Part model, mm, in its own coordinate system. A direction names the side the tool comes from. Coordinates: 2 decimals unless noted, no trailing zeros. Write each loop counter-clockwise with the first axis right and the second up, starting at its lowest first coordinate (ties: lowest second). Pieces come first, ordered by that corner, then holes. Notation, with made-up numbers: M 25,77 L 57,77 A14 cw 57,90 Z; hole C -7,86 d3. An arc over 180 degrees is marked long. Use a Markdown table: item, result. Add a question column.
Q1. Wall check: L1, parallel to X at y = -10.5, z = 0.5; L2, parallel to X at y = -56.9, z = -6; L3, parallel to Y at x = -12.5, z = 35.5. Give the ranges that are in metal, low to high. Write a range as from..to.
Q2. Mould opens along Y. For faces 6 (the flat face through (-39, -59, 9)), 7 (the flat face through (18.14, -46.86, 18.79)), 8 (the flat face through (12.606, 9, 2)), 9 (the flat face through (8.106, 9, 2)) say: released by +Y, released by -Y, zero draft, split by the parting line, or undercut.
Q3. Slice it at B-B on z = -6. Write the cut outline in (x, y), then the cut area to 3 significant figures.
Q4. Slice it at C-C on x = -11. Write the cut outline in (y, z).
Q5. Slice it at D-D on z = 29.5. Write the cut outline in (x, y), then the cut area to 3 significant figures.
Q6. Slice it at A-A on y = 1.5. Write the cut outline in (x, z).
Q7. Tool access for faces 1 (the flat face through (-4, -62.073, 29)), 2 (the flat face through (-4, -59, -15)), 3 (the flat face through (-22.394, 9, 2)), 4 (the flat face through (-5, -10, 0)), 5 (the cylindrical face through (-42.89, -59.59, -5.91)): list every direction of +Z, -Z, +X, -X, +Y, -Y with a clear straight run to the whole face (end or side of a thin tool).
Q8. Pin check, flat tips, straight feed: pin 1 Ø24 at (y, z) = (-48, 23.5) entering from -X; pin 2 Ø2 at (x, y) = (-15.5, 15.5) entering from +Z; pin 3 Ø12 at (x, y) = (11, -1.5) entering from -Z; pin 4 Ø6 at (y, z) = (-38.5, 18) entering from +X. Stop position of each tip, or through.
from build123d import *

# Parameters (mm, degrees)
ESQUISSE1_W             = 50
ESQUISSE1_H             = 95
BOSS_EXTRU_1_DEPTH      = 4
ESQUISSE2_W             = 50
ESQUISSE2_H             = 4
BOSS_EXTRU_2_DEPTH      = 5
ESQUISSE3_W             = 50
ESQUISSE3_H             = 5
BOSS_EXTRU_3_DEPTH      = 5
ESQUISSE4_W             = 50
ESQUISSE4_H             = 4
BOSS_EXTRU_4_DEPTH      = 40
ESQUISSE5_W             = 50
ESQUISSE5_H             = 5
BOSS_EXTRU_5_DEPTH      = 15
ENL_V_MAT_EXTRU_1_REACH = 21
BOSS_EXTRU_6_DEPTH      = 5
BOSS_EXTRU_7_DEPTH      = 5
BOSS_EXTRU_8_DEPTH      = 20
BOSS_EXTRU_9_DEPTH      = 20
ENL_V_MAT_EXTRU_2_REACH = 12
ESQUISSE12_R            = 1.5
ESQUISSE13_R            = 2
ENL_V_MAT_EXTRU_3_DEPTH = 3


with BuildPart() as part:
    # Esquisse1 → Boss.-Extru.1 (new body)
    with BuildSketch(Plane.XY):
        with Locations((-4.39396009, -13.572795505)):
            Rectangle(ESQUISSE1_W, ESQUISSE1_H)
    extrude(amount=BOSS_EXTRU_1_DEPTH)

    # Esquisse2 → Boss.-Extru.2 (add)
    with BuildSketch(Plane.XY.offset(4)):
        with Locations((-4.39396009, -59.072795505)):
            Rectangle(ESQUISSE2_W, ESQUISSE2_H)
    extrude(amount=BOSS_EXTRU_2_DEPTH)

    # Esquisse3 → Boss.-Extru.3 (add)
    with BuildSketch(Plane.XZ.offset(61.072795505)):
        with Locations((-4.39396009, 6.5)):
            Rectangle(ESQUISSE3_W, ESQUISSE3_H)
    extrude(amount=BOSS_EXTRU_3_DEPTH)

    # Esquisse4 → Boss.-Extru.4 (add)
    with BuildSketch(Plane.XY.offset(9)):
        with Locations((-4.39396009, -64.072795505)):
            Rectangle(ESQUISSE4_W, ESQUISSE4_H)
    extrude(amount=BOSS_EXTRU_4_DEPTH)

    # Esquisse5 → Boss.-Extru.5 (add)
    with BuildSketch(Plane(origin=(0, 0, 0), x_dir=(-1, 0, 0), z_dir=(0, 0, -1))):
        with Locations((4.39396009, -58.572795505)):
            Rectangle(ESQUISSE5_W, ESQUISSE5_H)
    extrude(amount=BOSS_EXTRU_5_DEPTH)

    # Esquisse6 → Enlèv. mat.-Extru.1 (cut, up to next)
    with BuildSketch(Plane.XY.offset(4), mode=Mode.PRIVATE) as enl_v_mat_extru_1_sk1:
        with BuildLine():
            Line((-17.89396009, 28.927204495), (-17.89396009, -11.072795505))
            ThreePointArc((-17.89396009, -11.072795505), (-20.14396009, -13.322795505), (-22.39396009, -11.072795505))
            Line((-22.39396009, -11.072795505), (-22.39396009, 28.927204495))
            ThreePointArc((-22.39396009, 28.927204495), (-20.14396009, 31.177204495), (-17.89396009, 28.927204495))
        make_face()
    enl_v_mat_extru_1_tool1 = extrude(enl_v_mat_extru_1_sk1.sketch, amount=-ENL_V_MAT_EXTRU_1_REACH, mode=Mode.PRIVATE) & part.part
    add(enl_v_mat_extru_1_tool1.solids().sort_by_distance((-20.14396, 8.927204, 4))[0], mode=Mode.SUBTRACT)
    # Esquisse6 → Enlèv. mat.-Extru.1 (cut, up to next)
    with BuildSketch(Plane.XY.offset(4), mode=Mode.PRIVATE) as enl_v_mat_extru_1_sk2:
        with BuildLine():
            Line((12.60603991, 28.927204495), (12.60603991, -11.072795505))
            ThreePointArc((12.60603991, -11.072795505), (10.35603991, -13.322795505), (8.10603991, -11.072795505))
            Line((8.10603991, -11.072795505), (8.10603991, 28.927204495))
            ThreePointArc((8.10603991, 28.927204495), (10.35603991, 31.177204495), (12.60603991, 28.927204495))
        make_face()
    enl_v_mat_extru_1_tool2 = extrude(enl_v_mat_extru_1_sk2.sketch, amount=-ENL_V_MAT_EXTRU_1_REACH, mode=Mode.PRIVATE) & part.part
    add(enl_v_mat_extru_1_tool2.solids().sort_by_distance((10.35604, 8.927204, 4))[0], mode=Mode.SUBTRACT)

    # Esquisse7 → Boss.-Extru.6 (add)
    with BuildSketch(Plane.ZY.offset(29.39396009)):
        Polygon((4, -32.072795505), (34, -62.072795505), (4, -62.072795505), align=None)
    extrude(amount=-BOSS_EXTRU_6_DEPTH)

    # Esquisse8 → Boss.-Extru.7 (add)
    with BuildSketch(Plane(origin=(20.60603991, 0, 0), x_dir=(0, 0, -1), z_dir=(1, 0, 0))):
        Polygon((-4, -32.072795505), (-34, -62.072795505), (-4, -62.072795505), align=None)
    extrude(amount=-BOSS_EXTRU_7_DEPTH)

    # Esquisse10 → Boss.-Extru.8 (add)
    with BuildSketch(Plane(origin=(20.60603991, 0, 0), x_dir=(0, 0, -1), z_dir=(1, 0, 0))):
        Polygon((-49, -62.072795505), (-49, -66.072795505), (-4, -66.072795505), (-4, -61.072795505), (15, -61.072795505), (15, -56.072795505), (0, -56.072795505), (-9, -56.072795505), (-9, -62.072795505), align=None)
    extrude(amount=BOSS_EXTRU_8_DEPTH)

    # Esquisse11 → Boss.-Extru.9 (add)
    with BuildSketch(Plane.ZY.offset(29.39396009)):
        Polygon((49, -66.072795505), (4, -66.072795505), (4, -61.072795505), (-15, -61.072795505), (-15, -56.072795505), (0, -56.072795505), (9, -56.072795505), (9, -62.072795505), (49, -62.072795505), align=None)
    extrude(amount=BOSS_EXTRU_9_DEPTH)

    # Esquisse12 → Enlèv. mat.-Extru.2 (cut, up to next)
    with BuildSketch(Plane(origin=(0, -56.072795505, 0), x_dir=(1, 0, 0), z_dir=(0, 1, 0)), mode=Mode.PRIVATE) as enl_v_mat_extru_2_sk1:
        with Locations((32.10603991, 6)):
            Circle(ESQUISSE12_R)
    enl_v_mat_extru_2_tool1 = extrude(enl_v_mat_extru_2_sk1.sketch, amount=-ENL_V_MAT_EXTRU_2_REACH, mode=Mode.PRIVATE) & part.part
    add(enl_v_mat_extru_2_tool1.solids().sort_by_distance((32.10604, -56.072796, -6))[0], mode=Mode.SUBTRACT)
    # Esquisse12 → Enlèv. mat.-Extru.2 (cut, up to next)
    with BuildSketch(Plane(origin=(0, -56.072795505, 0), x_dir=(1, 0, 0), z_dir=(0, 1, 0)), mode=Mode.PRIVATE) as enl_v_mat_extru_2_sk2:
        with Locations((-40.89396009, 6)):
            Circle(ESQUISSE12_R)
    enl_v_mat_extru_2_tool2 = extrude(enl_v_mat_extru_2_sk2.sketch, amount=-ENL_V_MAT_EXTRU_2_REACH, mode=Mode.PRIVATE) & part.part
    add(enl_v_mat_extru_2_tool2.solids().sort_by_distance((-40.89396, -56.072796, -6))[0], mode=Mode.SUBTRACT)

    # Esquisse13 → Enlèv. mat.-Extru.3 (cut)
    with BuildSketch(Plane.XZ.offset(61.072795505)):
        with Locations((32.10603991, -6)):
            Circle(ESQUISSE13_R)
        with Locations((-40.89396009, -6)):
            Circle(ESQUISSE13_R)
    extrude(amount=-ENL_V_MAT_EXTRU_3_DEPTH, mode=Mode.SUBTRACT)


solid = part.part
Recorded:
| question | item | result |
|---|---|---|
| 1 | L1 | -29.39..-22.39, -17.89..8.11, 12.61..20.61 |
| 1 | L2 | -49.39..-42.39, -39.39..30.61, 33.61..40.61 |
| 1 | L3 | -66.07..-62.07 |
| 2 | face 6 | zero draft |
| 2 | face 7 | released by +Y |
| 2 | face 8 | undercut |
| 2 | face 9 | undercut |
| 3 | outline | M -49.39,-61.07 L -42.89,-61.07 L -42.89,-58.07 L -42.39,-58.07 L -42.39,-56.07 L -49.39,-56.07 Z; M -39.39,-58.07 L -38.89,-58.07 L -38.89,-61.07 L 30.11,-61.07 L 30.11,-58.07 L 30.61,-58.07 L 30.61,-56.07 L -39.39,-56.07 Z; M 33.61,-58.07 L 34.11,-58.07 L 34.11,-61.07 L 40.61,-61.07 L 40.61,-56.07 L 33.61,-56.07 Z |
| 3 | area | 414 mm² |
| 4 | outline | M -66.07,4 L -61.07,4 L -61.07,-15 L -56.07,-15 L -56.07,0 L 33.93,0 L 33.93,4 L -57.07,4 L -57.07,9 L -62.07,9 L -62.07,49 L -66.07,49 Z |
| 5 | outline | M -49.39,-66.07 L 40.61,-66.07 L 40.61,-62.07 L 20.61,-62.07 L 20.61,-57.57 L 15.61,-57.57 L 15.61,-62.07 L -24.39,-62.07 L -24.39,-57.57 L -29.39,-57.57 L -29.39,-62.07 L -49.39,-62.07 Z |
| 5 | area | 405 mm² |
| 6 | outline | M -29.39,0 L -22.39,0 L -22.39,4 L -29.39,4 Z; M -17.89,0 L 8.11,0 L 8.11,4 L -17.89,4 Z; M 12.61,0 L 20.61,0 L 20.61,4 L 12.61,4 Z |
| 7 | face 1 | +Z, +Y |
| 7 | face 2 | -Z, +X, -X, +Y, -Y |
| 7 | face 3 | +Z, -Z |
| 7 | face 4 | -Z, +X, -X, +Y |
| 7 | face 5 | -Y |
| 8 | pin 1 | x = -29.39 |
| 8 | pin 2 | z = 4 |
| 8 | pin 3 | z = 0 |
| 8 | pin 4 | through |
